from build123d import *

# Parameters (mm, degrees)
SKETCH2_R          = 2.81
CUT_EXTRUDE1_DEPTH = 3.03


with BuildPart() as part:
    # Sketch1 → Revolve1 (revolve)
    with BuildSketch(Plane.XY):
        Polygon((0, 3.9), (-15, 3.9), (-15, 1.9), (-4.96, 1.9), (-4.96, 0), (0, 0), align=None)
    revolve(axis=Axis((0, 3.9, 0), (0, -1, 0)))

    # Sketch2 → Cut-Extrude1 (cut)
    with BuildSketch(Plane.XZ):
        Circle(SKETCH2_R)
    extrude(amount=-CUT_EXTRUDE1_DEPTH, mode=Mode.SUBTRACT)


solid = part.part
Source: CAD feature listing. Evaluate the final solid. Frame: model axes, mm. A direction names the side the tool comes from. Coordinates: 2 decimals unless noted, no trailing zeros. Loops run counter-clockwise (first coordinate to the right, second up) from the corner with the lowest first, then second, coordinate; pieces in that order, holes last. Notation, with made-up numbers: (15.25, 31.5) - (48.25, 31.5) arc R21 ccw to (48.25, 35.5) - close; hole circle Ø2 at (-37.75, -21.75). An arc over 180 degrees is marked (long way). Return JSON: item names as keys, results as strings.
Q1. Access query for faces 4 (the flat face through (-2.1, 0, 2.1)), 5 (the flat face through (4, 1.9, -4)). Directions: +Z, -Z, +X, -X, +Y, -Y. A direction counts if a zero-diameter tool reaches every point of the face in a straight line with its end or side. Return the directions, or none.
Results:
{"face 4": "+Z, -Z, +X, -X, -Y", "face 5": "-Y"}
Q2. Section D-D, the plane x = 4. Return loops of the section in (y, z), plus the area to 3 significant figures.
Results:
{"outline": "(0, -2.93) - (1.9, -2.93) - (1.9, -14.46) - (3.9, -14.46) - (3.9, 14.46) - (1.9, 14.46) - (1.9, 2.93) - (0, 2.93) - close", "area": "69.0 mm2"}
Q3. Material intervals for line 1 along Z through (x, y) = (0, 1.2); line 2 along Y through (x, z) = (-7.5, 8); line 3 along Z through (x, y) = (0, 2.2), sorted ascending.
Results:
{"line 1": "-4.96 to -2.81, 2.81 to 4.96", "line 2": "1.9 to 3.9", "line 3": "-15 to -2.81, 2.81 to 15"}
Q4. Contact query for flat-ended pins moving along their axis: P1, Ø2, axis at x = 5, y = 2, coming from the -Z side; P2, Ø2, axis at x = 10, z = 3, coming from the -Y side; P3, Ø1, axis at x = 1.5, y = 1, coming from the +Z side. Output: stop coordinate, or through.
Results:
{"P1": "z = -14.46", "P2": "y = 1.9", "P3": "z = 4.86"}
Q5. Section C-C, the plane y = 1.15. Return loops of the section in (x, z).
Results:
{"outline": "circle Ø9.92 at (0, 0); hole circle Ø5.62 at (0, 0)"}
Q6. Mould query, pull axis X, two halves, no side actions, for faces 1 (the cylindrical face through (1.08, 0.94, 4.84)), 2 (the flat face through (0, 3.9, 0)), 3 (the cylindrical face through (-0.609, 1.494, -2.743)). Classes: released by +X, released by -X, zero draft, split by the parting line, or undercut.
Results:
{"face 1": "split by the parting line", "face 2": "zero draft", "face 3": "undercut"}
Q7. Section A-A, the plane x = 0. Return loops of the section in (y, z).
Results:
{"outline": "(0, -4.96) - (1.9, -4.96) - (1.9, -15) - (3.9, -15) - (3.9, 15) - (1.9, 15) - (1.9, 4.96) - (0, 4.96) - (0, 2.81) - (3.03, 2.81) - (3.03, -2.81) - (0, -2.81) - close"}
Q8. Section B-B, the plane z = 0. Return loops of the section in (x, y).
Results:
{"outline": "(-15, 1.9) - (-4.96, 1.9) - (-4.96, 0) - (-2.81, 0) - (-2.81, 3.03) - (2.81, 3.03) - (2.81, 0) - (4.96, 0) - (4.96, 1.9) - (15, 1.9) - (15, 3.9) - (-15, 3.9) - close"}
